Work out the finished part from the listing and answer in its coordinate system (mm). A direction names the side the tool comes from. Coordinates: 2 decimals unless noted, no trailing zeros. Loops run counter-clockwise (first coordinate to the right, second up) from the corner with the lowest first, then second, coordinate; pieces in that order, holes last.
```python
from build123d import *

# Parameters (mm, degrees)
F1_DEPTH = 26
F3_DEPTH = 42.692334


with BuildPart() as f1:
    # F0 (on Front) → F1 (new body)
    with BuildSketch(Plane.XZ):
        with BuildLine():
            Line((-9.599707, 9.211308), (-9.599707, 4.211308))
            Line((-9.599707, 4.211308), (29.200293, 4.211308))
            Line((29.200293, 4.211308), (43.600293, 29.152839))
            Line((43.600293, 29.152839), (48.600293, 37.813093))
            Line((48.600293, 37.813093), (39.870873, 42.691334))
            Line((39.870873, 42.691334), (23.628611, 16.571015))
            ThreePointArc((23.628611, 16.571015), (21.811412, 14.840869), (19.382571, 14.211308))
            Line((19.382571, 14.211308), (-4.599707, 14.211308))
            ThreePointArc((-4.599707, 14.211308), (-8.135241, 12.746842), (-9.599707, 9.211308))
        make_face()
        Polygon((48.600293, 37.813093), (43.600293, 29.152839), (60.920801, 19.152839), (65.920801, 27.813093), align=None)
    extrude(amount=F1_DEPTH)

    # F2 (on Top) → F3 (cut, through all)
    with BuildSketch(Plane.XY):
        with BuildLine():
            Line((0.116861, -10.002277), (0, -10))
            ThreePointArc((0, -10), (-3, -13), (0, -16))
            ThreePointArc((0, -16), (2.12132, -15.12132), (3, -13))
            ThreePointArc((3, -13), (2.162242, -10.920407), (0.116861, -10.002277))
        make_face()
        with BuildLine():
            ThreePointArc((0.116861, -10.002277), (0.058442, -10.000569), (0, -10))
            Line((0, -10), (0.116861, -10.002277))
        make_face()
        with BuildLine():
            ThreePointArc((3, -13), (2.12132, -15.12132), (0, -16))
            Line((0, -16), (11.941272, -16.233806))
            ThreePointArc((11.941272, -16.233806), (9.000572, -13.175796), (12.058442, -10.23495))
            Line((12.058442, -10.23495), (0.116861, -10.002277))
            ThreePointArc((0.116861, -10.002277), (2.162242, -10.920407), (3, -13))
        make_face()
        with BuildLine():
            ThreePointArc((12.058442, -10.23495), (9.000572, -13.175796), (11.941272, -16.233806))
            ThreePointArc((11.941272, -16.233806), (14.100454, -15.376364), (15, -13.234381))
            ThreePointArc((15, -13.234381), (14.141883, -11.133824), (12.058442, -10.23495))
        make_face()
    extrude(amount=F3_DEPTH, mode=Mode.SUBTRACT)


solid = f1.part
```
1. Each of these flat-tipped pins is pushed along its axis until it touches: P1, Ø2, axis at x = 52, y = -14.5, coming from the -Z side; P2, Ø1.5, axis at x = 9, y = -11, coming from the -Z side; P3, Ø3, axis at y = -8.5, z = 9, coming from the +X side; P4, Ø2, axis at y = -22.5, z = 37, coming from the -X side. Where does it stop, or does it pass through?
2. A cutting plane is placed at B-B, the plane x = 5. Give the vertices of the cut face in (y, z).
3. For faces 4 (the flat face through (52.139, -12.818, 24.223)), 5 (the flat face through (28, 0, 21)), 6 (the flat face through (8, -10, 14.211)), determine the directions among +Z, -Z, +X, -X, +Y, -Y from which every point of the face is accessible in a straight line to the end or side of a thin tool.
4. A cutting plane is placed at C-C, the plane x = 24.5. Give the vertices of the cut face in (y, z), then the cut area to 3 significant figures.
5. Determine the mould class of faces 1 (the flat face through (-9.6, -13, 7)), 2 (the cylindrical face through (-3, -13, 9)), 3 (the flat face through (28, -26, 21)) for opening direction Y: released by +Y, released by -Y, zero draft, split by the parting line, or undercut.
6. A cutting plane is placed at A-A, the plane y = -14.75. Give the vertices of the cut face in (x, z).
7. A cutting plane is placed at D-D, the plane z = 33.5. Give the vertices of the cut face in (x, y), then the cut area to 3 significant figures.
8. Straight lines are drawn through the part: probe 1 along Z at (x, y) = (17, -21); probe 2 along X at (y, z) = (-20.5, 20); probe 3 along X at (y, z) = (-7, 24.5). For each, find the intervals that lie inside material, in ascending order.
Answers below:
1. P1: stops at z = 23.73
1. P2: passes through
1. P3: stops at x = 32.83
1. P4: stops at x = 35.71
2. outline: (-26, 4.21) - (-16.1, 4.21) - (-16.1, 14.21) - (-26, 14.21) - close; (-10.1, 4.21) - (0, 4.21) - (0, 14.21) - (-10.1, 14.21) - close
3. face 4: -Z, +Y, -Y
3. face 5: +Z, -Z, +X, -X, +Y
3. face 6: +Z, -X, +Y, -Y
4. outline: (-26, 4.21) - (0, 4.21) - (0, 17.97) - (-26, 17.97) - close
4. area: 358 mm2
5. face 1: zero draft
5. face 2: undercut
5. face 3: released by -Y
6. outline: (-9.6, 4.21) - (-2.44, 4.21) - (-2.44, 14.21) - (-4.6, 14.21) arc R5 ccw to (-9.6, 9.21) - close; (14.59, 4.21) - (29.2, 4.21) - (43.6, 29.15) - (60.92, 19.15) - (65.92, 27.81) - (48.6, 37.81) - (39.87, 42.69) - (23.63, 16.57) arc R5 cw to (19.38, 14.21) - (14.59, 14.21) - close
7. outline: (34.16, -26) - (56.07, -26) - (56.07, 0) - (34.16, 0) - close
7. area: 570 mm2
8. probe 1: z = 4.21 to 14.21
8. probe 2: x = 25.76 to 38.32, 59.45 to 61.41
8. probe 3: x = 28.56 to 40.91, 51.66 to 64.01
